Design review of the part shown in the three views and the two pictorial views. Dimensions are in mm from the part's minimum x, y and z. Give positions to 0.01 mm unless a question says otherwise; leave off trailing zeros. Loops run counter-clockwise (first coordinate to the right, second up) from the corner with the lowest first, then second, coordinate; pieces in that order, holes last. Notation, with made-up numbers: (5, 10) - (48, 10) arc R25 cw to (48, 30) - close; hole circle Ø10 at (15.5, 72.25). An arc over 180 degrees is marked (long way). Answer as a JSON object with one key per item and string values.
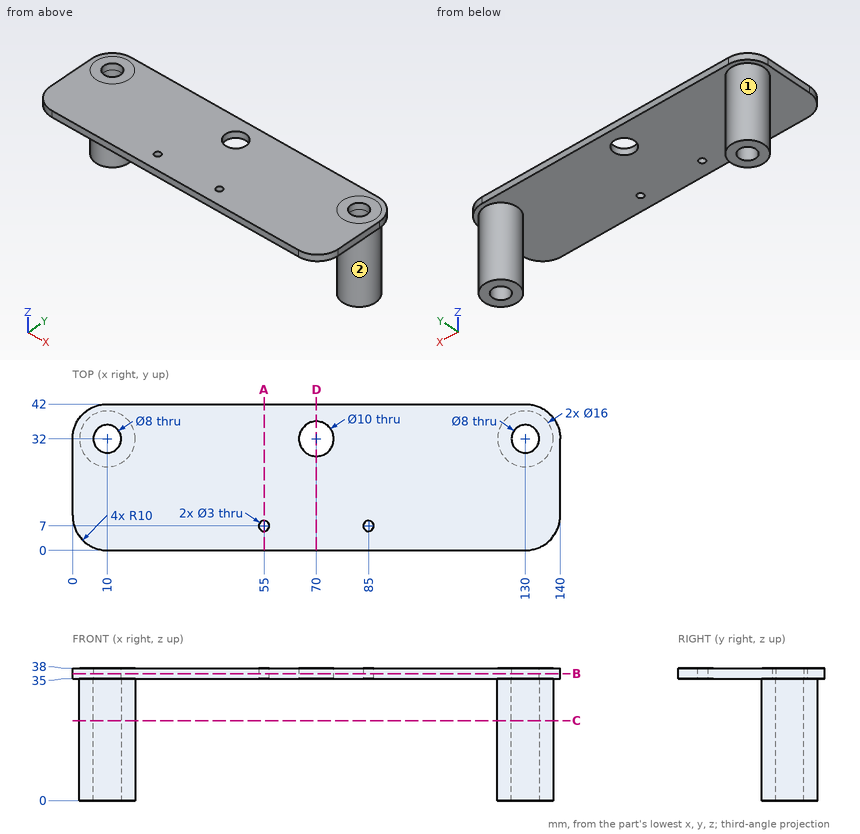
Q1. Consider section A-A, the plane x = 55. State the section outline as (y, z) points, plus the area to 3 significant figures.
Results:
{"outline": "(0, 35) - (5.5, 35) - (5.5, 38) - (0, 38) - close; (8.5, 35) - (42, 35) - (42, 38) - (8.5, 38) - close", "area": "117 mm^2"}
Q2. The part is to be moulded in two halves that separate along X. For the marked faces 1 and 2, say which applies: +X half, -X half, draft (parallel to the pull), parting line (faces both ways), or undercut.
Results:
{"face 1": "undercut", "face 2": "undercut"}
Q3. To check wall thickness, follow probe 1 along Y at (x, z) = (130, 8); probe 2 along X at (y, z) = (35.5, 10.5); probe 3 along X at (y, z) = (31, 25.5). State the ranges of each line that lie inside material, in increasing order. Write a range as [from, to].
Results:
{"probe 1": "y = [24, 28], [36, 40]", "probe 2": "x = [2.81, 8.06], [11.94, 17.19], [122.81, 128.06], [131.94, 137.19]", "probe 3": "x = [2.06, 6.13], [13.87, 17.94], [122.06, 126.13], [133.87, 137.94]"}
Q4. Consider section B-B, the plane z = 36.5. State the section outline as (x, y) points.
Results:
{"outline": "(0, 10) arc R10 ccw to (10, 0) - (130, 0) arc R10 ccw to (140, 10) - (140, 32) arc R10 ccw to (130, 42) - (10, 42) arc R10 ccw to (0, 32) - close; hole circle Ø8 at (10, 32); hole circle Ø3 at (55, 7); hole circle Ø10 at (70, 32); hole circle Ø3 at (85, 7); hole circle Ø8 at (130, 32)"}
Q5. Consider section D-D, the plane x = 70. State the section outline as (y, z) points, plus the area to 3 significant figures.
Results:
{"outline": "(0, 35) - (27, 35) - (27, 38) - (0, 38) - close; (37, 35) - (42, 35) - (42, 38) - (37, 38) - close", "area": "96.0 mm^2"}
Q6. Consider section C-C, the plane z = 23. State the section outline as (x, y) points.
Results:
{"outline": "circle Ø16 at (10, 32); circle Ø16 at (130, 32); hole circle Ø8 at (10, 32); hole circle Ø8 at (130, 32)"}
Q7. Clearance check with flat-ended pins moving along their axes: pin 1 Ø8 at (x, y) = (102.5, 5) entering from -Z; pin 2 Ø1 at (y, z) = (34.5, 4.5) entering from -X; pin 3 Ø1 at (y, z) = (37, 17) entering from -X. State where each tip first meets the part, or that it passes through.
Results:
{"pin 1": "stops at z = 35", "pin 2": "stops at x = 2.25", "pin 3": "stops at x = 3.39"}
